Design review of the part shown in the three views and the two pictorial views. Dimensions are in mm from the part's minimum x, y and z. Round coordinates to 2 decimals unless told otherwise and drop trailing zeros. Order: outer loops, then holes, each group sorted by start corner. A loop starts at its lowest first (then second) coordinate and runs counter-clockwise, first axis right, second up.
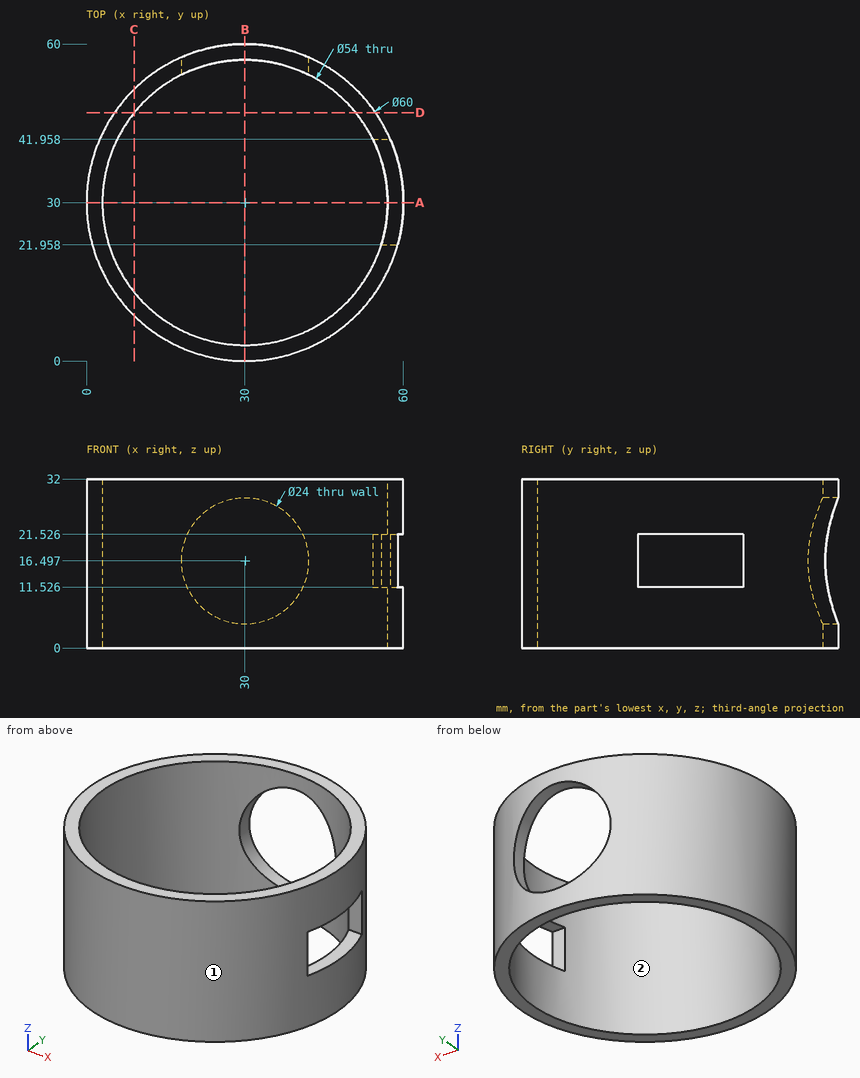
1) Take a section at C-C on x = 9. Give the boundary of the cut face in (y, z) (1 decimal), plus the area to 3 significant figures.
Results:
outline: (8.6, 0) - (13, 0) - (13, 32) - (8.6, 32) - close; (47, 0) - (51.4, 0) - (51.4, 32) - (47, 32) - close
area: 285 mm2
2) Clearance check with flat-ended pins moving along their axes: P1, Ø2, axis at x = 36, z = 19.5, coming from the -Y side; P2, Ø1.7, axis at x = 56.5, z = 17.5, coming from the -Y side; P3, Ø10, axis at y = 44.5, z = 23, coming from the -X side. State where each tip first meets the part, or that it passes through.
Results:
P1: stops at y = 0.42
P2: stops at y = 14.44
P3: stops at x = 1.54
3) The part is to be moulded in two halves that separate along Y. For the marked faces 1 and 2, say which applies: released by +Y, released by -Y, zero draft, split by the parting line, or undercut.
Results:
face 1: split by the parting line
face 2: undercut
4) To check wall thickness, follow line 1 along Z through (x, y) = (56, 40.5); line 2 along Z through (x, y) = (31.5, 57.5); line 3 along X through (y, z) = (37.5, 9). State the ranges of each line that lie inside material, in increasing order.
Results:
line 1: z = 0 to 11.53, 21.53 to 32
line 2: z = 0 to 4.59, 28.4 to 32
line 3: x = 0.95 to 4.06, 55.94 to 59.05
5) Take a section at A-A on y = 30. Give the boundary of the cut face in (x, z), plus the area to 3 significant figures.
Results:
outline: (0, 0) - (3, 0) - (3, 32) - (0, 32) - close; (57, 0) - (60, 0) - (60, 11.53) - (57, 11.53) - close; (57, 21.53) - (60, 21.53) - (60, 32) - (57, 32) - close
area: 162 mm2
6) Take a section at B-B on x = 30. Give the boundary of the cut face in (y, z), plus the area to 3 significant figures.
Results:
outline: (0, 0) - (3, 0) - (3, 32) - (0, 32) - close; (57, 0) - (60, 0) - (60, 4.5) - (57, 4.5) - close; (57, 28.5) - (60, 28.5) - (60, 32) - (57, 32) - close
area: 120 mm2
7) Take a section at D-D on y = 47. Give the boundary of the cut face in (x, z).
Results:
outline: (5.28, 0) - (9.02, 0) - (9.02, 32) - (5.28, 32) - close; (50.98, 0) - (54.72, 0) - (54.72, 32) - (50.98, 32) - close
